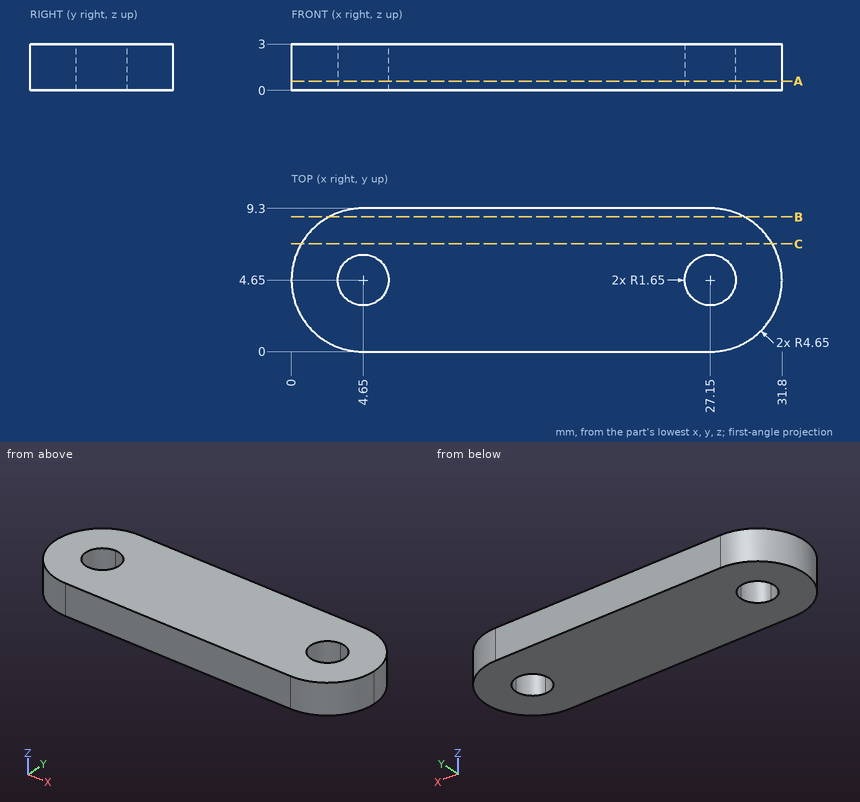
Can you work these out from the drawing? Everything is in mm from the part's minimum corner. Give positions to 0.01 mm unless a question says otherwise; leave off trailing zeros. Order: outer loops, then holes, each group sorted by start corner. A loop starts at its lowest first (then second) coordinate and runs counter-clockwise, first axis right, second up.
Item 1: If we section it at C-C, the plane y = 7: Write out the boundary of the cut face in (x, z).
Item 2: If we section it at A-A, the plane z = 0.6: Write out the boundary of the cut face in (x, y).
Item 3: I need wall thicknesses on line 1 (X direction, y = 4.5, z = 0.3); line 2 (Y direction, x = 6, z = 1.75); line 3 (Y direction, x = 28.5, z = 2.05). Which ranges of each line are inside material? Lowest first, please.
Item 4: I'm going to push a flat-ended pin straight in: pin 1 (5 mm diameter, centred on x = 8, y = 2, fed in from -Z). Where does the tip first touch, or does it pass through?
Item 5: If we section it at B-B, the plane y = 8.75: Write out the boundary of the cut face in (x, z).
Values:
1. outline: (0.64, 0) - (31.16, 0) - (31.16, 3) - (0.64, 3) - close
2. outline: (4.65, 0) - (27.15, 0) arc R4.65 ccw to (27.15, 9.3) - (4.65, 9.3) arc R4.65 ccw to start; hole circle Ø3.3 at (4.65, 4.65); hole circle Ø3.3 at (27.15, 4.65)
3. line 1: x = 0 to 3.01, 6.29 to 25.51, 28.79 to 31.8
3. line 2: y = 0 to 3.7, 5.6 to 9.3
3. line 3: y = 0.2 to 3.7, 5.6 to 9.1
4. pin 1: stops at z = 0
5. outline: (2.46, 0) - (29.34, 0) - (29.34, 3) - (2.46, 3) - close
